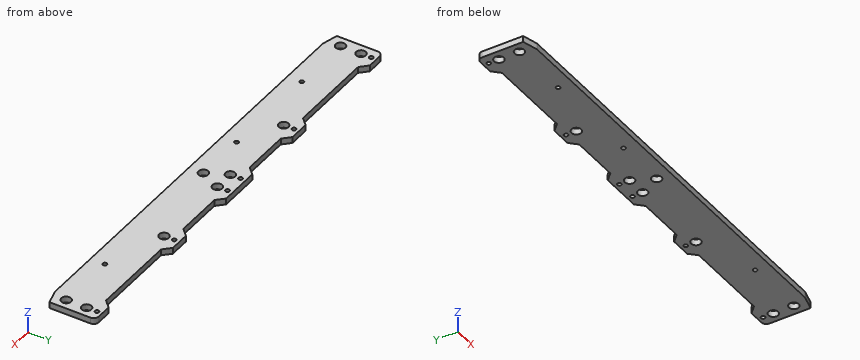
from build123d import *

# Parameters (mm, degrees)
CROQUIS1_R              = 4.75
SALIENTE_EXTRUIR1_DEPTH = 6
SALIENTE_EXTRUIR2_DEPTH = 6
CROQUIS3_R              = 2
CORTAR_EXTRUIR1_DEPTH   = 225.635259922
SALIENTE_EXTRUIR3_DEPTH = 6
REDONDEO3_R             = 5


with BuildPart() as part:
    # Croquis1 → Saliente-Extruir1 (new body)
    with BuildSketch(Plane.XY):
        Polygon((-220, 0), (220, 0), (220, 38), (108.6, 38), (101.6, 45), (81.6, 45), (74.6, 38), (27, 38), (20, 45), (-20, 45), (-27, 38), (-74.6, 38), (-81.6, 45), (-101.6, 45), (-108.6, 38), (-220, 38), align=None)
        with Locations((-210, 10)):
            Circle(CROQUIS1_R, mode=Mode.SUBTRACT)
        with Locations((-210, 30)):
            Circle(CROQUIS1_R, mode=Mode.SUBTRACT)
        with Locations(Location((210, 10, 0), (0, 0, 180))):
            Circle(CROQUIS1_R, mode=Mode.SUBTRACT)
        with Locations(Location((210, 30, 0), (0, 0, 180))):
            Circle(CROQUIS1_R, mode=Mode.SUBTRACT)
        with Locations((-91.6, 30)):
            Circle(CROQUIS1_R, mode=Mode.SUBTRACT)
        with Locations((-10, 30)):
            Circle(CROQUIS1_R, mode=Mode.SUBTRACT)
        with Locations(Location((10, 30, 0), (0, 0, 180))):
            Circle(CROQUIS1_R, mode=Mode.SUBTRACT)
        with Locations(Location((91.6, 30, 0), (0, 0, 180))):
            Circle(CROQUIS1_R, mode=Mode.SUBTRACT)
        with Locations((0, 10)):
            Circle(CROQUIS1_R, mode=Mode.SUBTRACT)
    extrude(amount=SALIENTE_EXTRUIR1_DEPTH)

    # Croquis2 → Saliente-Extruir2 (add)
    with BuildSketch(Plane.XY.offset(6)):
        Polygon((-220, 38), (-220, 45), (-200, 45), (-193, 38), align=None)
        Polygon((200, 45), (193, 38), (220, 38), (220, 45), align=None)
    extrude(amount=-SALIENTE_EXTRUIR2_DEPTH)

    # Croquis3 → Cortar-Extruir1 (cut, through all)
    with BuildSketch(Plane.XY.offset(6)):
        with Locations((-91.6, 40)):
            Circle(CROQUIS3_R)
        with Locations((-210, 40)):
            Circle(CROQUIS3_R)
        with Locations((-10, 40)):
            Circle(CROQUIS3_R)
        with Locations(Location((10, 40, 0), (0, 0, 180))):
            Circle(CROQUIS3_R)
        with Locations(Location((91.6, 40, 0), (0, 0, 180))):
            Circle(CROQUIS3_R)
        with Locations(Location((210, 40, 0), (0, 0, 180))):
            Circle(CROQUIS3_R)
        with Locations((-150.8, 10)):
            Circle(CROQUIS3_R)
        with Locations((-50.8, 10)):
            Circle(CROQUIS3_R)
        with Locations(Location((150.8, 10, 0), (0, 0, 180))):
            Circle(CROQUIS3_R)
    extrude(amount=-CORTAR_EXTRUIR1_DEPTH, mode=Mode.SUBTRACT)

    # Croquis4 → Saliente-Extruir3 (add)
    with BuildSketch(Plane.XY.offset(6)):
        Polygon((220, 0), (-220, 0), (-205.07179677, -4), (205.07179677, -4), align=None)
    extrude(amount=-SALIENTE_EXTRUIR3_DEPTH)

    # Redondeo3
    redondeo3_edges = [part.edges().sort_by_distance(p)[0] for p in [
        (-220, 45, 3),
        (220, 45, 3),
    ]]
    fillet(redondeo3_edges, radius=REDONDEO3_R)


solid = part.part
Build history of the part. All positions in model axes, mm. Round coordinates to 2 decimals unless told otherwise and drop trailing zeros. Loops run counter-clockwise (first coordinate to the right, second up) from the corner with the lowest first, then second, coordinate; pieces in that order, holes last. Notation, with made-up numbers: (-36, -12.75) -> (0, -12.75) arc R14 ccw to (0, -4.75) -> close; hole circle Ø3 at (-10.5, 14.25). An arc over 180 degrees is marked (long way). Answer in a Markdown table with one row per item.
Item 1: Drill centre lines: L1, parallel to Y at x = 9.5, z = 4.15; L2, parallel to Y at x = -10, z = 2.05; L3, parallel to Y at x = 210, z = 2.3. Where is each one in solid material? Low to high. Write a range as [from, to].
Answers below:
| item | result |
|---|---|
| L1 | y = [-4, 25.28], [34.72, 38.06], [41.94, 45] |
| L2 | y = [-4, 25.25], [34.75, 38], [42, 45] |
| L3 | y = [-2.68, 5.25], [14.75, 25.25], [34.75, 38], [42, 45] |
Item 2: Saw through at C-C (x = 53). Write the cut outline in (y, z).
Answers below:
| item | result |
|---|---|
| outline | (-4, 0) -> (38, 0) -> (38, 6) -> (-4, 6) -> close |
Item 3: Saw through at B-B (z = 4.4). State how many separate pieces and enclosed holes the cut face has, and give its area (3 significant figures).
Answers below:
| item | result |
|---|---|
| separate pieces | 1 |
| enclosed holes | 18 |
| area | 18,700 mm² |
Item 4: Pin check, flat tips, straight feed: pin 1 (12.5 mm diameter, centred on x = -91.6, y = 30, fed in from -Z); pin 2 (1.8 mm diameter, centred on x = 48, z = 1.5, fed in from +Y). Stop position of each tip, or through.
Answers below:
| item | result |
|---|---|
| pin 1 | stops at z = 0 |
| pin 2 | stops at y = 38 |
Item 5: Saw through at A-A (y = 30). Write the cut outline in (x, z), and give its area (3 significant figures).
Answers below:
| item | result |
|---|---|
| outline | (-220, 0) -> (-214.75, 0) -> (-214.75, 6) -> (-220, 6) -> close; (-205.25, 0) -> (-96.35, 0) -> (-96.35, 6) -> (-205.25, 6) -> close; (-86.85, 0) -> (-14.75, 0) -> (-14.75, 6) -> (-86.85, 6) -> close; (-5.25, 0) -> (5.25, 0) -> (5.25, 6) -> (-5.25, 6) -> close; (14.75, 0) -> (86.85, 0) -> (86.85, 6) -> (14.75, 6) -> close; (96.35, 0) -> (205.25, 0) -> (205.25, 6) -> (96.35, 6) -> close; (214.75, 0) -> (220, 0) -> (220, 6) -> (214.75, 6) -> close |
| area | 2,300 mm² |
